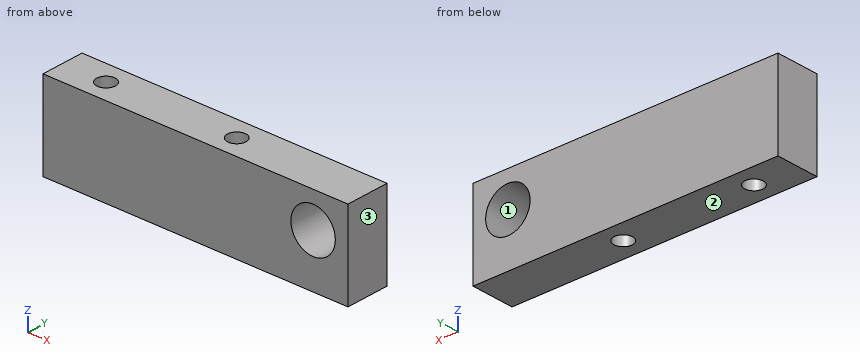
```python
from build123d import *

# Parameters (mm, degrees)
F0_W     = 44.45
F0_H     = 12.7
F0_R     = 3.2385
F1_DEPTH = 6.35
F3_D     = 2.7051


with BuildPart() as f1:
    # F0 (on Front) → F1 (new body)
    with BuildSketch(Plane.XZ):
        Rectangle(F0_W, F0_H)
        with Locations((17.145, 1.27)):
            Circle(F0_R, mode=Mode.SUBTRACT)
    extrude(amount=F1_DEPTH)

    # F3 (through all)
    with Locations(Plane(origin=(0, 0, -6.35), x_dir=(1, 0, 0), z_dir=(0, 0, -1))):
        with Locations((-15.875, 3.175), (3.175, 3.175)):
            Hole(F3_D / 2)


solid = f1.part
```
CAD build for the part. Positions are in the model's coordinates, mm. Face numbers are marked on the shaded views. Give positions to 0.01 mm unless a question says otherwise; leave off trailing zeros. Order: outer loops, then holes, each group sorted by start corner. A loop starts at its lowest first (then second) coordinate and runs counter-clockwise, first axis right, second up. Notation, with made-up numbers: M 60.5,82.5 L 73.5,82.5 A24 ccw 73.5,105.5 Z; hole C -35.5,44.25 d1. An arc over 180 degrees is marked long. Put each result on its own line as item: value. Start each with the question number.
(1) Flat gauge pins, fed straight in: pin 1 Ø2.5 at (x, y) = (3.175, -3.175) entering from -Z; pin 2 Ø1 at (x, z) = (-11, -0.5) entering from +Y. Where does each tip first touch, or does it go through?
(2) Mould opens along X. For the marked faces 1, 2 and 3 say: +X half, -X half, draft (parallel to the pull), parting line (faces both ways), or undercut.
(3) Saw through at C-C, the plane x = 18. Write the cut outline in (y, z).
(4) Saw through at A-A, the plane z = 2.25. Write the cut outline in (x, y) (3 decimals), then the cut area to 3 significant figures.
(5) Saw through at B-B, the plane y = -2.25. Give the number of separate pieces and of enclosed holes in the cut face, then the cut area to 3 significant figures.
(6) Drill centre lines: line 1 along X through (y, z) = (-3, 3.25) (3 decimals); line 2 along X through (y, z) = (-4, -2.75) (3 decimals); line 3 along X through (y, z) = (-2.25, -4) (3 decimals). Where is each one in solid material? Low to high.
Check result:
1. pin 1: passes through
1. pin 2: stops at y = 0
2. face 1: undercut
2. face 2: draft
2. face 3: +X half
3. outline: M -6.35,-6.35 L 0,-6.35 L 0,-1.85 L -6.35,-1.85 Z; M -6.35,4.39 L 0,4.39 L 0,6.35 L -6.35,6.35 Z
4. outline: M -22.225,-6.35 L 14.058,-6.35 L 14.058,0 L -22.225,0 Z; M 20.232,-6.35 L 22.225,-6.35 L 22.225,0 L 20.232,0 Z; hole C -15.875,-3.175 d2.705; hole C 3.175,-3.175 d2.705
4. area: 232 mm2
5. separate pieces: 3
5. enclosed holes: 1
5. area: 481 mm2
6. line 1: x = -22.225 to -17.216, -14.534 to 1.834, 4.516 to 14.582, 19.708 to 22.225
6. line 2: x = -22.225 to -16.947, -14.803 to 2.103, 4.247 to 22.225
6. line 3: x = -22.225 to -16.862, -14.888 to 2.188, 4.162 to 22.225
